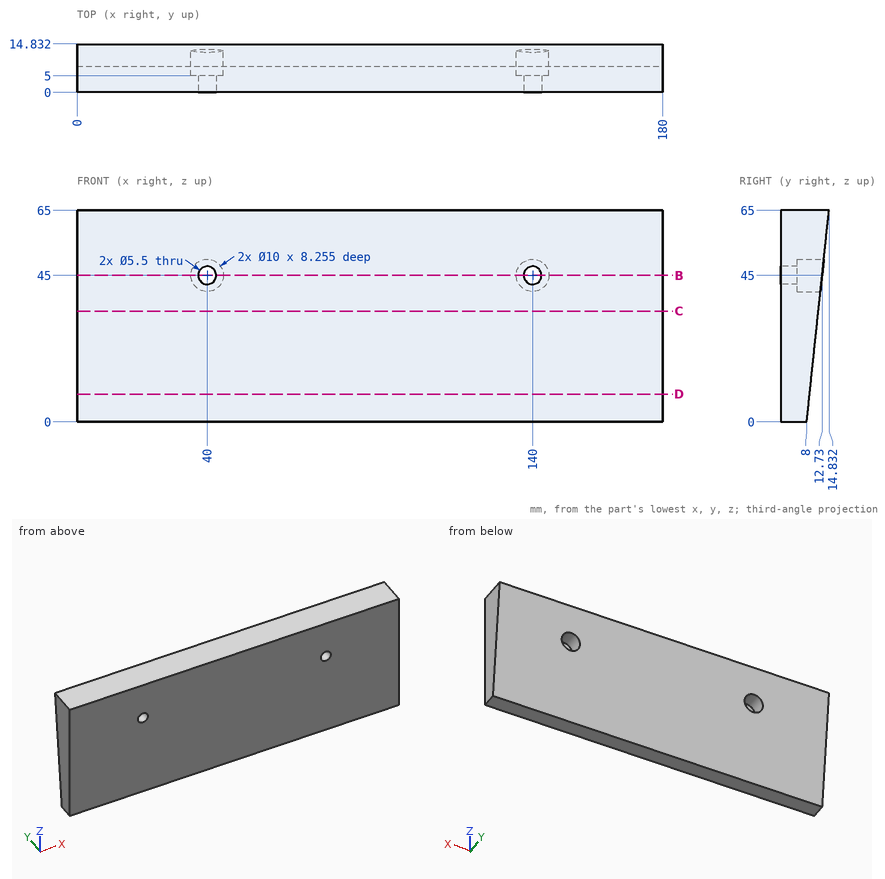
Part print with two shaded views. Sizes in mm from the minimum x, y, z corner. Round coordinates to 2 decimals unless told otherwise and drop trailing zeros. Order: outer loops, then holes, each group sorted by start corner. A loop starts at its lowest first (then second) coordinate and runs counter-clockwise, first axis right, second up. Notation, with made-up numbers: (-19, 24.5) - (28, 24.5) arc R10 ccw to (28, 36.5) - close; hole circle Ø6 at (18, 46). An arc over 180 degrees is marked (long way). Answer as CSV lines item,"result". Start each with the question number.
1. Saw through at B-B, the plane z = 45. Write the cut outline in (x, y), and give its area (3 significant figures).
2. Saw through at C-C, the plane z = 34. Write the cut outline in (x, y), and give its area (3 significant figures).
3. Drill centre lines: L1, parallel to X at y = 8.5, z = 45; L2, parallel to X at y = 2.9, z = 45; L3, parallel to Z at x = 140, y = 2.2. Where is each one in solid material? Low to high. Write a range as [from, to].
4. Saw through at D-D, the plane z = 8.5. Write the cut outline in (x, y), and give its area (3 significant figures).
5. Pin check, flat tips, straight feed: pin 1 (5 mm diameter, centred on x = 40, z = 45, fed in from +Y); pin 2 (1.5 mm diameter, centred on x = 137, z = 36, fed in from +Y); pin 3 (8 mm diameter, centred on x = 38, z = 44.5, fed in from +Y); pin 4 (11 mm diameter, centred on x = 140.5, z = 44, fed in from +Y). Stop position of each tip, or through.
Model answer:
1,outline,"(0, 0) - (37.25, 0) - (37.25, 5) - (35, 5) - (35, 12.73) - (0, 12.73) - close; (42.75, 0) - (137.25, 0) - (137.25, 5) - (135, 5) - (135, 12.73) - (45, 12.73) - (45, 5) - (42.75, 5) - close; (142.75, 0) - (180, 0) - (180, 12.73) - (145, 12.73) - (145, 5) - (142.75, 5) - close"
1,area,"2,080 mm²"
2,outline,"(0, 0) - (180, 0) - (180, 11.57) - (0, 11.57) - close"
2,area,"2,080 mm²"
3,L1,"x = [0, 35], [45, 135], [145, 180]"
3,L2,"x = [0, 37.25], [42.75, 137.25], [142.75, 180]"
3,L3,"z = [0, 42.25], [47.75, 65]"
4,outline,"(0, 0) - (180, 0) - (180, 8.89) - (0, 8.89) - close"
4,area,"1,600 mm²"
5,pin 1,"passes through"
5,pin 2,"stops at y = 11.86"
5,pin 3,"stops at y = 13.04"
5,pin 4,"stops at y = 13.12"
